Here's the drawing with two shaded views (mm, measured from the low corner). I have some questions. Give positions to 0.01 mm unless a question says otherwise; leave off trailing zeros. Loops run counter-clockwise (first coordinate to the right, second up) from the corner with the lowest first, then second, coordinate; pieces in that order, holes last. Notation, with made-up numbers: M 20.5,19.25 L 64.5,19.25 A14 cw 64.5,45.25 Z; hole C -9.5,65.25 d1. An arc over 180 degrees is marked long. Put each result on its own line as item: value. Start each with the question number.
1) Please list where these lines run through material, in increasing order: line 1 along X through (y, z) = (2.05, 4) (1 decimal); line 2 along Y through (x, z) = (14.25, 4); line 3 along X through (y, z) = (2.05, 22). Write a range as from..to.
2) Imagine slicing it at D-D (x = 9.5). Write out the boundary of the cut face in (y, z).
3) Imagine slicing it at B-B (z = 11.25). Write out the boundary of the cut face in (x, y) (1 decimal).
4) For P1, Ø1.6, axis at x = 3.5, z = 22.495, coming from the +Y side; P2, Ø2, axis at x = 9.5, y = 4.5, coming from the +Z side; P3, Ø3, axis at x = 13, z = 13.5, coming from the +Y side (1 decimal); P4, Ø2.5, axis at x = 15.5, z = 3.255, coming from the +Y side, each with a flat end and sliding along its axis, tell me the tip position at first contact or that it passes through.
5) Imagine slicing it at A-A (x = 15.5). State how many separate pieces and enclosed holes the cut face has.
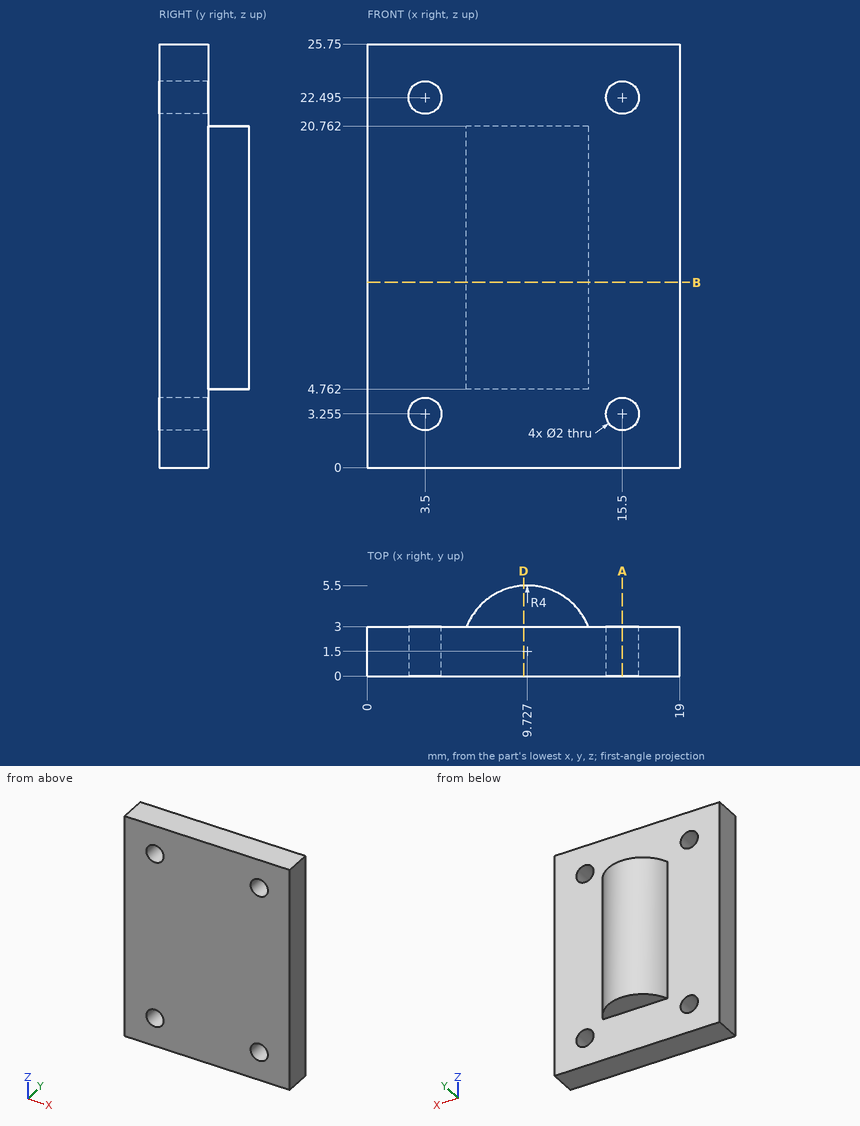
Recorded:
1. line 1: 0..2.8, 4.2..14.8, 16.2..19
1. line 2: 0..3
1. line 3: 0..2.63, 4.37..14.63, 16.37..19
2. outline: M 0,0 L 3,0 L 3,4.76 L 5.49,4.76 L 5.49,20.76 L 3,20.76 L 3,25.75 L 0,25.75 Z
3. outline: M 0,0 L 19,0 L 19,3 L 13.4,3 A4 ccw 6,3 L 0,3 Z
4. P1: through
4. P2: z = 20.76
4. P3: y = 5.1
4. P4: y = 3
5. separate pieces: 3
5. enclosed holes: 0
